```python
from build123d import *

# Parameters (mm, degrees)
BOSS_EXTRUDE1_DEPTH = 5
BOSS_EXTRUDE2_START = 5
BOSS_EXTRUDE2_DEPTH = 3
BOSS_EXTRUDE3_START = 8
BOSS_EXTRUDE3_DEPTH = 100
CHAMFER1_SIZE       = 14
CHAMFER1_SIZE2      = 88.392521205
CUT_EXTRUDE1_REACH  = 228.845
CUT_EXTRUDE2_REACH  = 243.541
CUT_EXTRUDE3_START  = 5
CUT_EXTRUDE3_DEPTH  = 25.406962
BOSS_EXTRUDE4_DEPTH = 4
BOSS_EXTRUDE5_START = -108
BOSS_EXTRUDE5_DEPTH = 8


with BuildPart() as part:
    # Sketch1 → Boss-Extrude1 (new body)
    # profile 1 of 5: a face of its own
    with BuildSketch(Plane(origin=(0, 0, 0), x_dir=(1, 0, 0), z_dir=(0, 1, 0))):
        with BuildLine():
            Line((-67.63171498, -190.215666308), (-67.63171498, -178.666752182))
            Line((-67.63171498, -178.666752182), (-84.707225068, -178.666752182))
            Line((-84.707225068, -178.666752182), (-84.707225068, -190.215666308))
            ThreePointArc((-84.707225068, -190.215666308), (-76.169470024, -198.753421352), (-67.63171498, -190.215666308))
        make_face()
    # profile 2 of 5: a face of its own
    with BuildSketch(Plane(origin=(0, 0, 0), x_dir=(1, 0, 0), z_dir=(0, 1, 0))):
        with BuildLine():
            Line((-84.707225068, -178.666752182), (-67.63171498, -178.666752182))
            Line((-67.63171498, -178.666752182), (-67.63171498, -106.004837653))
            ThreePointArc((-67.63171498, -106.004837653), (-75.871331662, -98.476802493), (-84.707225068, -105.29512957))
            Line((-84.707225068, -105.29512957), (-84.707225068, -178.666752182))
        make_face()
        with BuildLine():
            ThreePointArc((-80.169470024, -160.215666308), (-76.169470024, -156.215666308), (-72.169470024, -160.215666308))
            Line((-72.169470024, -160.215666308), (-72.169470024, -164.215666308))
            ThreePointArc((-72.169470024, -164.215666308), (-76.169470024, -168.215666308), (-80.169470024, -164.215666308))
            Line((-80.169470024, -164.215666308), (-80.169470024, -160.215666308))
        make_face(mode=Mode.SUBTRACT)
        with BuildLine():
            ThreePointArc((-80.169470024, -110.004837653), (-76.169470024, -106.004837653), (-72.169470024, -110.004837653))
            Line((-72.169470024, -110.004837653), (-72.169470024, -114.004837653))
            ThreePointArc((-72.169470024, -114.004837653), (-76.169470024, -118.004837653), (-80.169470024, -114.004837653))
            Line((-80.169470024, -114.004837653), (-80.169470024, -110.004837653))
        make_face(mode=Mode.SUBTRACT)
    # profile 3 of 5: a face of its own
    with BuildSketch(Plane(origin=(0, 0, 0), x_dir=(1, 0, 0), z_dir=(0, 1, 0))):
        with BuildLine():
            Line((-80.169470024, -160.215666308), (-80.169470024, -164.215666308))
            ThreePointArc((-80.169470024, -164.215666308), (-76.169470024, -168.215666308), (-72.169470024, -164.215666308))
            Line((-72.169470024, -164.215666308), (-72.169470024, -160.215666308))
            ThreePointArc((-72.169470024, -160.215666308), (-76.169470024, -156.215666308), (-80.169470024, -160.215666308))
        make_face()
        with BuildLine():
            ThreePointArc((-74.169470024, -160.294008998), (-76.169470024, -158.294008998), (-78.169470024, -160.294008998))
            Line((-78.169470024, -160.294008998), (-78.169470024, -164.215666308))
            ThreePointArc((-78.169470024, -164.215666308), (-76.169470024, -166.215666308), (-74.169470024, -164.215666308))
            Line((-74.169470024, -164.215666308), (-74.169470024, -160.294008998))
        make_face(mode=Mode.SUBTRACT)
    # profile 4 of 5: a face of its own
    with BuildSketch(Plane(origin=(0, 0, 0), x_dir=(1, 0, 0), z_dir=(0, 1, 0))):
        with BuildLine():
            Line((-80.169470024, -110.004837653), (-80.169470024, -114.004837653))
            ThreePointArc((-80.169470024, -114.004837653), (-76.169470024, -118.004837653), (-72.169470024, -114.004837653))
            Line((-72.169470024, -114.004837653), (-72.169470024, -110.004837653))
            ThreePointArc((-72.169470024, -110.004837653), (-76.169470024, -106.004837653), (-80.169470024, -110.004837653))
        make_face()
        with BuildLine():
            ThreePointArc((-74.169470024, -109.794008998), (-76.169470024, -107.794008998), (-78.169470024, -109.794008998))
            Line((-78.169470024, -109.794008998), (-78.169470024, -114.215666308))
            ThreePointArc((-78.169470024, -114.215666308), (-76.169470024, -116.215666308), (-74.169470024, -114.215666308))
            Line((-74.169470024, -114.215666308), (-74.169470024, -109.794008998))
        make_face(mode=Mode.SUBTRACT)
    # profile 5 of 5: a face of its own
    with BuildSketch(Plane(origin=(0, 0, 0), x_dir=(1, 0, 0), z_dir=(0, 1, 0))):
        with BuildLine():
            Line((-74.169470024, -164.215666308), (-74.169470024, -160.294008998))
            ThreePointArc((-74.169470024, -160.294008998), (-76.169470024, -158.294008998), (-78.169470024, -160.294008998))
            Line((-78.169470024, -160.294008998), (-78.169470024, -164.215666308))
            ThreePointArc((-78.169470024, -164.215666308), (-76.169470024, -166.215666308), (-74.169470024, -164.215666308))
        make_face()
    extrude(amount=BOSS_EXTRUDE1_DEPTH)

    # Sketch1<3> → Boss-Extrude2 (add)
    with BuildSketch(Plane(origin=(0, 0, 0), x_dir=(1, 0, 0), z_dir=(0, 1, 0)).offset(BOSS_EXTRUDE2_START)):
        with BuildLine():
            Line((-67.63171498, -190.215666308), (-67.63171498, -106.004837653))
            ThreePointArc((-67.63171498, -106.004837653), (-75.871331662, -98.476802493), (-84.707225068, -105.29512957))
            Line((-84.707225068, -105.29512957), (-84.707225068, -190.215666308))
            ThreePointArc((-84.707225068, -190.215666308), (-76.169470024, -198.753421352), (-67.63171498, -190.215666308))
        make_face()
        with BuildLine():
            Line((-72.169470024, -110.004837653), (-72.169470024, -114.004837653))
            ThreePointArc((-72.169470024, -114.004837653), (-76.169470024, -118.004837653), (-80.169470024, -114.004837653))
            Line((-80.169470024, -114.004837653), (-80.169470024, -110.004837653))
            ThreePointArc((-80.169470024, -110.004837653), (-76.169470024, -106.004837653), (-72.169470024, -110.004837653))
        make_face(mode=Mode.SUBTRACT)
    extrude(amount=BOSS_EXTRUDE2_DEPTH)

    # Sketch1<4> → Boss-Extrude3 (add)
    with BuildSketch(Plane(origin=(0, 0, 0), x_dir=(1, 0, 0), z_dir=(0, 1, 0)).offset(BOSS_EXTRUDE3_START)):
        with BuildLine():
            Line((-67.63171498, -190.215666308), (-67.63171498, -178.666752182))
            Line((-67.63171498, -178.666752182), (-84.707225068, -178.666752182))
            Line((-84.707225068, -178.666752182), (-84.707225068, -190.215666308))
            ThreePointArc((-84.707225068, -190.215666308), (-76.169470024, -198.753421352), (-67.63171498, -190.215666308))
        make_face()
    extrude(amount=BOSS_EXTRUDE3_DEPTH)

    # Chamfer1
    chamfer1_edges = [part.edges().sort_by_distance(p)[0] for p in [
        (-76.169470024, 8, 178.666752182),
    ]]
    chamfer1_side = [part.faces().sort_by_distance(p)[0] for p in [
        (-76.174011802, 8, 141.227226291),
    ]]
    chamfer(chamfer1_edges, length=CHAMFER1_SIZE, length2=CHAMFER1_SIZE2, reference=chamfer1_side[0])

    # Fillet1
    # an asymmetric fillet: 31, 15 mm, written as the material it adds along each edge
    with BuildSketch(Plane(origin=(-67.63171498, 8, 164.666752182), x_dir=(0, 0.9876883405951381, 0.15643446504022812), z_dir=(-1, 0, 0))) as fillet1_piece_1:
        with BuildLine():
            Bezier((10.277059237, 0), (0, 0), (-4.538265872, 28.653483024), weights=[1, 0.760405966, 1])
            Line((-4.538265872, 28.653483024), (0, 0))
            Line((0, 0), (10.277059237, 0))
        make_face()
    extrude(amount=17.075510088)

    # Sketch2 → Cut-Extrude1 (cut, up to next)
    with BuildSketch(Plane.ZY.offset(84.707225068), mode=Mode.PRIVATE) as cut_extrude1_sk1:
        Polygon((190.215666308, 91.769109668), (182.636112577, 91.769109668), (190.215666308, 64.31043598), align=None)
    cut_extrude1_tool1 = extrude(cut_extrude1_sk1.sketch, amount=-CUT_EXTRUDE1_REACH, mode=Mode.PRIVATE) & part.part
    # Sketch2 → Cut-Extrude1 (cut, up to next)
    with BuildSketch(Plane.ZY.offset(84.707225068), mode=Mode.PRIVATE) as cut_extrude1_sk2:
        Polygon((176.154286922, 48.567173756), (180.595955478, 76.61076533), (186.42899162, 55.479252617), align=None)
    cut_extrude1_tool2 = extrude(cut_extrude1_sk2.sketch, amount=-CUT_EXTRUDE1_REACH, mode=Mode.PRIVATE) & part.part
    # Sketch2 → Cut-Extrude1 (cut, up to next)
    with BuildSketch(Plane.ZY.offset(84.707225068), mode=Mode.PRIVATE) as cut_extrude1_sk3:
        Polygon((190.215666308, 12.025794409), (190.215666308, 50.795315392), (178.946314561, 43.21410987), align=None)
    cut_extrude1_tool3 = extrude(cut_extrude1_sk3.sketch, amount=-CUT_EXTRUDE1_REACH, mode=Mode.PRIVATE) & part.part
    # Sketch2 → Cut-Extrude1 (cut, up to next)
    with BuildSketch(Plane.ZY.offset(84.707225068), mode=Mode.PRIVATE) as cut_extrude1_sk4:
        Polygon((174.47148672, 37.942391428), (185.290645631, 8), (169.729077811, 8), align=None)
    cut_extrude1_tool4 = extrude(cut_extrude1_sk4.sketch, amount=-CUT_EXTRUDE1_REACH, mode=Mode.PRIVATE) & part.part
    # Sketch2 → Cut-Extrude1 (cut, up to next)
    with BuildSketch(Plane.ZY.offset(84.707225068), mode=Mode.PRIVATE) as cut_extrude1_sk5:
        Polygon((185.02175896, 104.554188767), (183.698567215, 96.199884882), (190.215666308, 96.199884882), (190.215666308, 104.554188767), align=None)
    cut_extrude1_tool5 = extrude(cut_extrude1_sk5.sketch, amount=-CUT_EXTRUDE1_REACH, mode=Mode.PRIVATE) & part.part
    add(cut_extrude1_tool1.solids().sort_by_distance((-84.707225, 82.616218, 187.689148))[0], mode=Mode.SUBTRACT)
    add(cut_extrude1_tool2.solids().sort_by_distance((-84.707225, 60.219064, 181.059745))[0], mode=Mode.SUBTRACT)
    add(cut_extrude1_tool3.solids().sort_by_distance((-84.707225, 35.345073, 186.459216))[0], mode=Mode.SUBTRACT)
    add(cut_extrude1_tool4.solids().sort_by_distance((-84.707225, 17.980797, 176.49707))[0], mode=Mode.SUBTRACT)
    add(cut_extrude1_tool5.solids().sort_by_distance((-84.707225, 100.219716, 187.275456))[0], mode=Mode.SUBTRACT)

    # Sketch1<5> → Cut-Extrude2 (cut, up to next)
    with BuildSketch(Plane(origin=(0, 0, 0), x_dir=(1, 0, 0), z_dir=(0, 1, 0)), mode=Mode.PRIVATE) as cut_extrude2_sk1:
        with BuildLine():
            Line((-74.169470024, -164.215666308), (-74.169470024, -160.294008998))
            ThreePointArc((-74.169470024, -160.294008998), (-76.169470024, -158.294008998), (-78.169470024, -160.294008998))
            Line((-78.169470024, -160.294008998), (-78.169470024, -164.215666308))
            ThreePointArc((-78.169470024, -164.215666308), (-76.169470024, -166.215666308), (-74.169470024, -164.215666308))
        make_face()
    cut_extrude2_tool1 = extrude(cut_extrude2_sk1.sketch, amount=CUT_EXTRUDE2_REACH, mode=Mode.PRIVATE) & part.part
    add(cut_extrude2_tool1.solids().sort_by_distance((-76.16947, 0, 162.254838))[0], mode=Mode.SUBTRACT)

    # Sketch1<6> → Cut-Extrude3 (cut)
    with BuildSketch(Plane(origin=(0, 0, 0), x_dir=(1, 0, 0), z_dir=(0, 1, 0)).offset(CUT_EXTRUDE3_START)):
        with BuildLine():
            Line((-80.169470024, -160.215666308), (-80.169470024, -164.215666308))
            ThreePointArc((-80.169470024, -164.215666308), (-76.169470024, -168.215666308), (-72.169470024, -164.215666308))
            Line((-72.169470024, -164.215666308), (-72.169470024, -160.215666308))
            ThreePointArc((-72.169470024, -160.215666308), (-76.169470024, -156.215666308), (-80.169470024, -160.215666308))
        make_face()
        with BuildLine():
            ThreePointArc((-74.169470024, -160.294008998), (-76.169470024, -158.294008998), (-78.169470024, -160.294008998))
            Line((-78.169470024, -160.294008998), (-78.169470024, -164.215666308))
            ThreePointArc((-78.169470024, -164.215666308), (-76.169470024, -166.215666308), (-74.169470024, -164.215666308))
            Line((-74.169470024, -164.215666308), (-74.169470024, -160.294008998))
        make_face(mode=Mode.SUBTRACT)
    extrude(amount=CUT_EXTRUDE3_DEPTH, mode=Mode.SUBTRACT)

    # Sketch4 → Boss-Extrude4 (add)
    with BuildSketch(Plane(origin=(0, 108, 0), x_dir=(1, 0, 0), z_dir=(0, 1, 0))):
        with BuildLine():
            Line((-67.63171498, -178.666752182), (-67.63171498, -198.666752182))
            ThreePointArc((-67.63171498, -198.666752182), (-68.803287856, -201.495179307), (-71.63171498, -202.666752182))
            Line((-71.63171498, -202.666752182), (-80.707225068, -202.666752182))
            ThreePointArc((-80.707225068, -202.666752182), (-83.535652193, -201.495179307), (-84.707225068, -198.666752182))
            Line((-84.707225068, -198.666752182), (-84.707225068, -178.666752182))
            Line((-84.707225068, -178.666752182), (-67.63171498, -178.666752182))
        make_face()
    extrude(amount=BOSS_EXTRUDE4_DEPTH)

    # Sketch4<2> → Boss-Extrude5 (add)
    with BuildSketch(Plane(origin=(0, 108, 0), x_dir=(1, 0, 0), z_dir=(0, 1, 0)).offset(BOSS_EXTRUDE5_START)):
        with BuildLine():
            Line((-67.63171498, -178.666752182), (-67.63171498, -198.666752182))
            ThreePointArc((-67.63171498, -198.666752182), (-68.803287856, -201.495179307), (-71.63171498, -202.666752182))
            Line((-71.63171498, -202.666752182), (-80.707225068, -202.666752182))
            ThreePointArc((-80.707225068, -202.666752182), (-83.535652193, -201.495179307), (-84.707225068, -198.666752182))
            Line((-84.707225068, -198.666752182), (-84.707225068, -178.666752182))
            Line((-84.707225068, -178.666752182), (-67.63171498, -178.666752182))
        make_face()
    extrude(amount=BOSS_EXTRUDE5_DEPTH)


solid = part.part
```
Source: CAD feature listing. Evaluate the final solid. Frame: model axes, mm. A direction names the side the tool comes from. Coordinates: 2 decimals unless noted, no trailing zeros. Loops run counter-clockwise (first coordinate to the right, second up) from the corner with the lowest first, then second, coordinate; pieces in that order, holes last. Notation, with made-up numbers: (56, 59) -> (82, 59) arc R30 cw to (82, 96) -> close; hole circle Ø10 at (-1.75, 16). An arc over 180 degrees is marked (long way). One line per item, written item: value. Start each with the question number.
Q1. Section query B-B, the plane y = 85.5. Return the cut outline in (x, z), and give its area (3 significant figures).
Q2. Contact query for flat-ended pins moving along their axis: P1, Ø5, axis at x = -82.5, y = 46, coming from the +Z side; P2, Ø6, axis at x = -72, z = 133, coming from the +Y side; P3, Ø4, axis at x = -70.5, z = 143, coming from the +Y side. Output: stop coordinate, or through.
Q3. Mould query, pull axis Z, two halves, no side actions, for faces 6 (the face through (-78.169, 2, 162)), 7 (the face through (-76, 8, 199)), 8 (the face through (-83.5, 3.94, 201.53)). Classes: pulls with the +Z half, pulls with the -Z half, needs draft (parallel to the pull), parting line crosses it, or undercut.
Q4. Set-up query: faces 1 (the face through (-76, 110, 202.667)), 2 (the face through (-74.169, 2, 162)), 3 (the face through (-84.707, 35, 169.5)), 4 (the face through (-76.29, 52.07, 181.36)), 5 (the face through (-76.082, 7.747, 156.217)). Return all of +Z, -Z, +X, -X, +Y, -Y with unobstructed straight access to the full face (end or side cutting, diameter ignored); none if empty.
Q5. Section query D-D, the plane z = 133. Return the cut outline in (x, y), and give its area (3 significant figures).
Q6. Section query A-A, the plane y = 70. Return the cut outline in (x, z).
Q7. Section query C-C, the plane x = -83. Give the number of separate pieces and of enclosed holes in the cut face, and give its area (3 significant figures).
Q8. Line query: line 1 along Z through (x, y) = (-73.25, 23); line 2 along Z through (x, y) = (-75.75, 34); line 3 along Y through (x, z) = (-72, 198). Output: solid intervals per line, ascending.
Results:
1. outline: (-84.71, 176.94) -> (-67.63, 176.94) -> (-67.63, 184.37) -> (-84.71, 184.37) -> close; (-84.71, 190.22) -> (-67.63, 190.22) arc R8.54 ccw to start
1. area: 241 mm^2
2. P1: z = 197.85
2. P2: y = 8
2. P3: y = 8.48
3. face 6: undercut
3. face 7: needs draft
3. face 8: pulls with the +Z half
4. face 1: +Z, +X, -X, +Y, -Y
4. face 2: +Y, -Y
4. face 3: +Z, -Z, -X, +Y, -Y
4. face 4: +X, -X
4. face 5: +Y
5. outline: (-84.71, 0) -> (-67.63, 0) -> (-67.63, 8) -> (-84.71, 8) -> close
5. area: 137 mm^2
6. outline: (-84.71, 174.49) -> (-67.63, 174.49) -> (-67.63, 179.55) -> (-84.71, 179.55) -> close; (-84.71, 182.42) -> (-67.63, 182.42) -> (-67.63, 188.65) -> (-84.71, 188.65) -> close; (-84.71, 190.22) -> (-67.63, 190.22) arc R8.54 ccw to start
7. separate pieces: 1
7. enclosed holes: 5
7. area: 2,510 mm^2
8. line 1: 167.04 to 172.1, 179.87 to 186.25, 190.22 to 198.24
8. line 2: 168.78 to 173.85, 175.9 to 182.28, 190.22 to 198.74
8. line 3: 0 to 8, 108 to 112
